Design review of the part built by this model. Coordinates are the model's own, in mm. Face numbers are marked on the shaded views. A direction names the side the tool comes from. Coordinates: 2 decimals unless noted, no trailing zeros. Write each loop counter-clockwise with the first axis right and the second up, starting at its lowest first coordinate (ties: lowest second). Pieces come first, ordered by that corner, then holes. Notation, with made-up numbers: (79.5, 20.25) -> (138.5, 20.25) arc R17 ccw to (138.5, 50.25) -> close; hole circle Ø9 at (-37, 19.5). An arc over 180 degrees is marked (long way). One line per question, with ' | ' between items. Start each with the question number.
Q1. Add section A-A on y = 0. State the section outline as (x, z) points, and give its area (3 significant figures).
Q2. For the marked faces 1 and 2, list the 3-axis set-ups (+Z, -Z, +X, -X, +Y, -Y) from which the entire face can be reached by the end or side of a thin tool; tool diameter is ignored.
Q3. For P1, Ø4, axis at x = 0.5, z = 21, coming from the -Y side; P2, Ø6, axis at x = -3, y = -19, coming from the +Z side; P3, Ø6, axis at x = -1.5, y = 18, coming from the -Z side; P4, Ø6, axis at y = 7, z = 17.5, coming from the -X side, all flat-tipped, find the tip position at first contact; note any pin that passes through.
Q4. Wall thickness on probe 1 along Z at (x, y) = (-30.5, 12.5); probe 2 along X at (y, z) = (-5.5, 16); probe 3 along Y at (x, z) = (-18.5, 10.5): over which ranges is each line inside the solid? List them lowest first.
Q5. Add section C-C on z = 14. State the section outline as (x, y) points, and give its area (3 significant figures).
from build123d import *

# Parameters (mm, degrees)
F0_R     = 41
F0_R_2   = 13.5
F1_DEPTH = 15
F2_DEPTH = 35
F3_R     = 5


with BuildPart() as f1:
    # F0 (on Top) → F1 (new body)
    with BuildSketch(Plane.XY):
        Circle(F0_R)
        Circle(F0_R_2, mode=Mode.SUBTRACT)
    extrude(amount=F1_DEPTH)

    # F0 (on Top) → F2 (join)
    with BuildSketch(Plane.XY):
        Circle(F0_R_2)
    extrude(amount=F2_DEPTH)

    # F3
    f3_edges = [f1.edges().sort_by_distance(p)[0] for p in [
        (-41, 0, 15),
        (-13.5, 0, 15),
    ]]
    fillet(f3_edges, radius=F3_R)


solid = f1.part
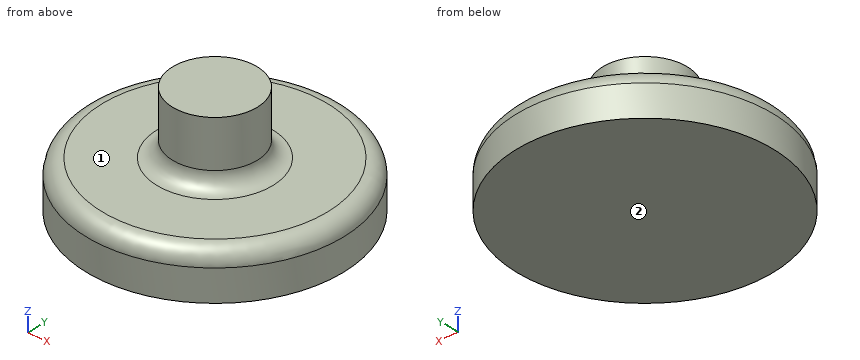
Output values:
1) outline: (-41, 0) -> (41, 0) -> (41, 10) arc R5 ccw to (36, 15) -> (18.5, 15) arc R5 cw to (13.5, 20) -> (13.5, 35) -> (-13.5, 35) -> (-13.5, 20) arc R5 cw to (-18.5, 15) -> (-36, 15) arc R5 ccw to (-41, 10) -> close | area: 1,770 mm2
2) face 1: +Z | face 2: -Z, +X, -X, +Y, -Y
3) P1: stops at y = -13.6 | P2: stops at z = 15.54 | P3: stops at z = 0 | P4: stops at x = -37.56
4) probe 1: z = 0 to 15 | probe 2: x = -14.49 to 14.49 | probe 3: y = -36.56 to 36.56
5) outline: circle Ø78 at (0, 0) | area: 4,780 mm2
